Geometry check sheet. Reference: the model listing, model coordinates, mm. A direction names the side the tool comes from. Coordinates: 2 decimals unless noted, no trailing zeros. Loops run counter-clockwise (first coordinate to the right, second up) from the corner with the lowest first, then second, coordinate; pieces in that order, holes last. Notation, with made-up numbers: M 0.5,-21.5 L 5.5,-21.5 A16 ccw 5.5,-9.5 Z; hole C 59,-25 d7. An arc over 180 degrees is marked long. Use CSV: the item, a comma, the result in double quotes.
```python
from build123d import *

# Parameters (mm, degrees)
SKETCH1_R           = 5
BOSS_EXTRUDE1_DEPTH = 110
SKETCH2_R           = 12.5
BOSS_EXTRUDE2_DEPTH = 5
FILLET1_R           = 1


with BuildPart() as part:
    # Sketch1 → Boss-Extrude1 (new, symmetric)
    with BuildSketch(Plane.XY):
        Circle(SKETCH1_R)
    extrude(amount=BOSS_EXTRUDE1_DEPTH, both=True)

    # Sketch2 → Boss-Extrude2 (add)
    with BuildSketch(Plane.XY.offset(110)):
        Circle(SKETCH2_R)
    extrude(amount=BOSS_EXTRUDE2_DEPTH)

    # Fillet1
    fillet1_edges = [part.edges().sort_by_distance(p)[0] for p in [
        (-12.5, 0, 115),
    ]]
    fillet(fillet1_edges, radius=FILLET1_R)


solid = part.part
```
1. Section check A-A, the plane y = 0. Record the cut outline in (x, z), plus the area to 3 significant figures.
The answers:
outline,"M -12.5,110 L -5,110 L -5,-110 L 5,-110 L 5,110 L 12.5,110 L 12.5,114 A1 ccw 11.5,115 L -11.5,115 A1 ccw -12.5,114 Z"
area,"2,320 mm^2"
2. Gauge pin test, flat ends, axial feed: P1, Ø2, axis at x = -8, y = 3, coming from the -Z side; P2, Ø8, axis at y = -3.5, z = -1, coming from the -X side; P3, Ø10, axis at x = 1.5, z = 0.5, coming from the +Y side; P4, Ø1.5, axis at x = 6, z = 79, coming from the +Y side. Record the tip position at first contact, or that the pin passes through.
The answers:
P1,"z = 110"
P2,"x = -5"
P3,"y = 5"
P4,"through"
3. Section check C-C, the plane z = 69.5. Record the cut outline in (x, y), plus the area to 3 significant figures.
The answers:
outline,"C 0,0 d10"
area,"78.5 mm^2"
4. Set-up check for faces 1 (the flat face through (0, 0, 115)), 2 (the flat face through (-0.2, -5.4, 110)): record each of +Z, -Z, +X, -X, +Y, -Y from which the full face is reachable in a straight line by a thin tool's end or side.
The answers:
face 1,"+Z, +X, -X, +Y, -Y"
face 2,"-Z"
5. Thickness scan on line 1 (Z direction, x = -10, y = 6); line 2 (Y direction, x = -4, z = -5.5); line 3 (Y direction, x = -2.5, z = -101). Record the ranges inside material, lowest first. Write a range as [from, to].
The answers:
line 1,"[110, 114.99]"
line 2,"[-3, 3]"
line 3,"[-4.33, 4.33]"
